Read the model definition and answer for the solid it produces. Units are mm, in the model's axes. A direction names the side the tool comes from. Give positions to 0.01 mm unless a question says otherwise; leave off trailing zeros. Order: outer loops, then holes, each group sorted by start corner. A loop starts at its lowest first (then second) coordinate and runs counter-clockwise, first axis right, second up.
Item 1: A cutting plane is placed at C-C (z = 5.5). Write down the section's boundary in (x, y).
Item 2: Which of the six approach directions +Z, -Z, +X, -X, +Y, -Y give full straight-line access (tool end or side, diameter ignored) to faces 1 (the face through (1, 0, 7)), 2 (the face through (-1.5, 0.07, 3.45))?
Item 3: Given pin 1 Ø0.8 at (x, y) = (0.5, 0.5) entering from +Z, flat-ended and moving along its own axis, determine where the tip first touches the part or whether it passes through.
Item 4: A cutting plane is placed at A-A (x = 0). Write down the section's boundary in (y, z).
Item 5: Find the intervals of material crossed by line 1 along Z through (x, y) = (-0.4, -0.8); line 2 along X through (y, z) = (1.3, 4.5); line 3 along X through (y, z) = (1.2, 4.75), in increasing order.
from build123d import *

# Parameters (mm, degrees)
F0_R     = 1.5
F1_DEPTH = 7
F5_SIZE  = 0.2


with BuildPart() as f1:
    # F0 (on Top) → F1 (new body)
    with BuildSketch(Plane.XY):
        Circle(F0_R)
    extrude(amount=F1_DEPTH)

    # F3 (on face) → F4 (revolve)
    with BuildSketch(Plane.XY.offset(7)):
        with BuildLine():
            Line((0, -0.75), (0, 0.75))
            ThreePointArc((0, 0.75), (-0.75, 0), (0, -0.75))
        make_face()
    revolve(axis=Axis((0, 0, 7), (0, 1, 0)))

    # F5
    f5_edges = [f1.edges().sort_by_distance(p)[0] for p in [
        (-1.5, 0, 7),
        (-1.5, 0, 0),
    ]]
    chamfer(f5_edges, length=F5_SIZE)


solid = f1.part
Response values:
1. outline: circle Ø3 at (0, 0)
2. face 1: +Z
2. face 2: +Z, -Z
3. pin 1: stops at z = 7.68
4. outline: (-1.5, 0.2) - (-1.3, 0) - (1.3, 0) - (1.5, 0.2) - (1.5, 6.8) - (1.3, 7) - (0.75, 7) arc R0.75 ccw to (-0.75, 7) - (-1.3, 7) - (-1.5, 6.8) - close
5. line 1: z = 0 to 7
5. line 2: x = -0.75 to 0.75
5. line 3: x = -0.9 to 0.9
